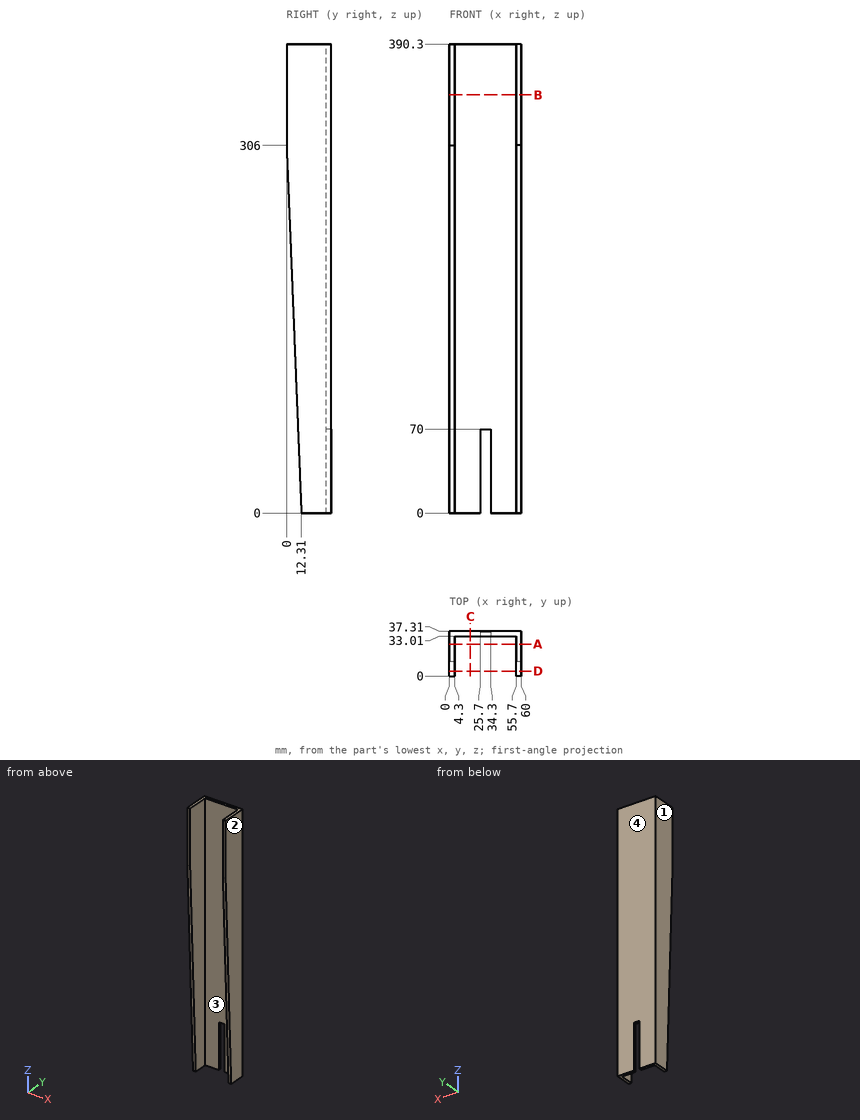
Can you work these out from the drawing? Everything is in mm from the part's minimum corner. Coordinates: 2 decimals unless noted, no trailing zeros. Order: outer loops, then holes, each group sorted by start corner. A loop starts at its lowest first (then second) coordinate and runs counter-clockwise, first axis right, second up. Notation, with made-up numbers: (7, -39) -> (15, -39) arc R9 cw to (15, -24) -> close; hole circle Ø2 at (19.5, 78). An arc over 180 degrees is marked (long way). Use one line per item in the form item = value.
Q1. Imagine slicing it at D-D, the plane y = 4. List the corners of the cut face in (x, z) for me.
From the geometry:
outline = (0, 206.57) -> (4.3, 206.57) -> (4.3, 390.3) -> (0, 390.3) -> close; (55.7, 206.57) -> (60, 206.57) -> (60, 390.3) -> (55.7, 390.3) -> close
Q2. Imagine slicing it at B-B, the plane z = 348. List the corners of the cut face in (x, y) for me.
From the geometry:
outline = (0, 0) -> (4.3, 0) -> (4.3, 33.01) -> (55.7, 33.01) -> (55.7, 0) -> (60, 0) -> (60, 37.31) -> (0, 37.31) -> close
Q3. Will these pins go through, and if not, where does the flat tip stop? P1, Ø3.5, axis at x = 29.5, y = 35, coming from the -Z side; P2, Ø1, axis at x = 27, z = 171.5, coming from the -Y side.
From the geometry:
P1 = 70
P2 = 33.01
Q4. Imagine slicing it at C-C, the plane x = 17.5. List the corners of the cut face in (y, z) for me.
From the geometry:
outline = (33.01, 0) -> (37.31, 0) -> (37.31, 390.3) -> (33.01, 390.3) -> close
Q5. Imagine slicing it at A-A, the plane y = 26.5. List the corners of the cut face in (x, z) for me, then the cut area to 3 significant figures.
From the geometry:
outline = (0, 0) -> (4.3, 0) -> (4.3, 390.3) -> (0, 390.3) -> close; (55.7, 0) -> (60, 0) -> (60, 390.3) -> (55.7, 390.3) -> close
area = 3,360 mm²
Q6. We'd pull the mould along X, two halves only. Please class the marked faces 1, 2, 3 and 4: released by +X, released by -X, zero draft, split by the parting line, or undercut.
From the geometry:
face_1 = released by -X
face_2 = released by +X
face_3 = undercut
face_4 = zero draft
Q7. I need wall thicknesses on L1, parallel to X at y = 11.5, z = 327; L2, parallel to Y at x = 25.5, z = 241.5; L3, parallel to Y at x = 4, z = 277.5. Which ranges of each line are inside material? Lowest first, please.
From the geometry:
L1 = 0 to 4.3, 55.7 to 60
L2 = 33.01 to 37.31
L3 = 1.15 to 37.31
